Build history of the part. All positions in model axes, mm. Round coordinates to 2 decimals unless told otherwise and drop trailing zeros. Write each loop counter-clockwise with the first axis right and the second up, starting at its lowest first coordinate (ties: lowest second). Pieces come first, ordered by that corner, then holes. Notation, with made-up numbers: M 39,40.25 L 82,40.25 A10 cw 82,45.25 Z; hole C 23,38.25 d8. An arc over 180 degrees is marked long. Use a Markdown table: item, result.
from build123d import *

# Parameters (mm, degrees)
SKETCH_1_R          = 1.5
EXTRUDE_2_DEPTH     = 3
SKETCH_2_R          = 1.5
CUT_EXTRUDE_1_DEPTH = 10


with BuildPart() as part:
    # 草图1 → 凸台-拉伸2 (new body)
    with BuildSketch(Plane(origin=(0, 0, 0), x_dir=(1, 0, 0), z_dir=(0, 1, 0))):
        with BuildLine():
            Line((-60, 65), (60, 65))
            ThreePointArc((60, 65), (125, 0), (60, -65))
            Line((60, -65), (-60, -65))
            ThreePointArc((-60, -65), (-125, 0), (-60, 65))
        make_face()
        with Locations((-122, 0)):
            Circle(SKETCH_1_R, mode=Mode.SUBTRACT)
        with Locations((122, 0)):
            Circle(SKETCH_1_R, mode=Mode.SUBTRACT)
        with Locations((-30, 60)):
            Circle(SKETCH_1_R, mode=Mode.SUBTRACT)
        with Locations((30, 60)):
            Circle(SKETCH_1_R, mode=Mode.SUBTRACT)
        with Locations((30, -60)):
            Circle(SKETCH_1_R, mode=Mode.SUBTRACT)
        with Locations((-30, -60)):
            Circle(SKETCH_1_R, mode=Mode.SUBTRACT)
    extrude(amount=EXTRUDE_2_DEPTH)

    # 草图2 → 切除-拉伸1 (cut)
    with BuildSketch(Plane(origin=(0, 3, 0), x_dir=(1, 0, 0), z_dir=(0, 1, 0))):
        with Locations((-10, 44)):
            Circle(SKETCH_2_R)
        with Locations((12, 44)):
            Circle(SKETCH_2_R)
        with Locations((-10, -44)):
            Circle(SKETCH_2_R)
        with Locations((12, -44)):
            Circle(SKETCH_2_R)
    extrude(amount=-CUT_EXTRUDE_1_DEPTH, mode=Mode.SUBTRACT)


solid = part.part
Q1. Cut at C-C on x = -89.5. Give the cut face in (y, z).
Response values:
| item | result |
|---|---|
| outline | M 0,-57.92 L 3,-57.92 L 3,57.92 L 0,57.92 Z |
Q2. Cut at B-B on z = 34.5. Give the cut face in (x, y).
Response values:
| item | result |
|---|---|
| outline | M -115.09,0 L 115.09,0 L 115.09,3 L -115.09,3 Z |
Q3. Drop a flat-ended pin along its axis: P1, Ø2.5, axis at x = -10, z = -44, coming from the -Y side. Give the stop position or say it passes through.
Response values:
| item | result |
|---|---|
| P1 | passes through |
Q4. Drill centre lines: L1, parallel to Z at x = 12, y = 1.35; L2, parallel to X at y = 1.7, z = 44; L3, parallel to Z at x = -30, y = 1.15. Where is each one in solid material? Low to high.
Response values:
| item | result |
|---|---|
| L1 | z = -65 to -45.5, -42.5 to 42.5, 45.5 to 65 |
| L2 | x = -107.84 to -11.5, -8.5 to 10.5, 13.5 to 107.84 |
| L3 | z = -65 to -61.5, -58.5 to 58.5, 61.5 to 65 |
Q5. Cut at A-A on y = 0.75. Count the separate pieces of the cut face and the enclosed holes in it, and give its area (3 significant figures).
Response values:
| item | result |
|---|---|
| separate pieces | 1 |
| enclosed holes | 10 |
| area | 28,800 mm2 |
